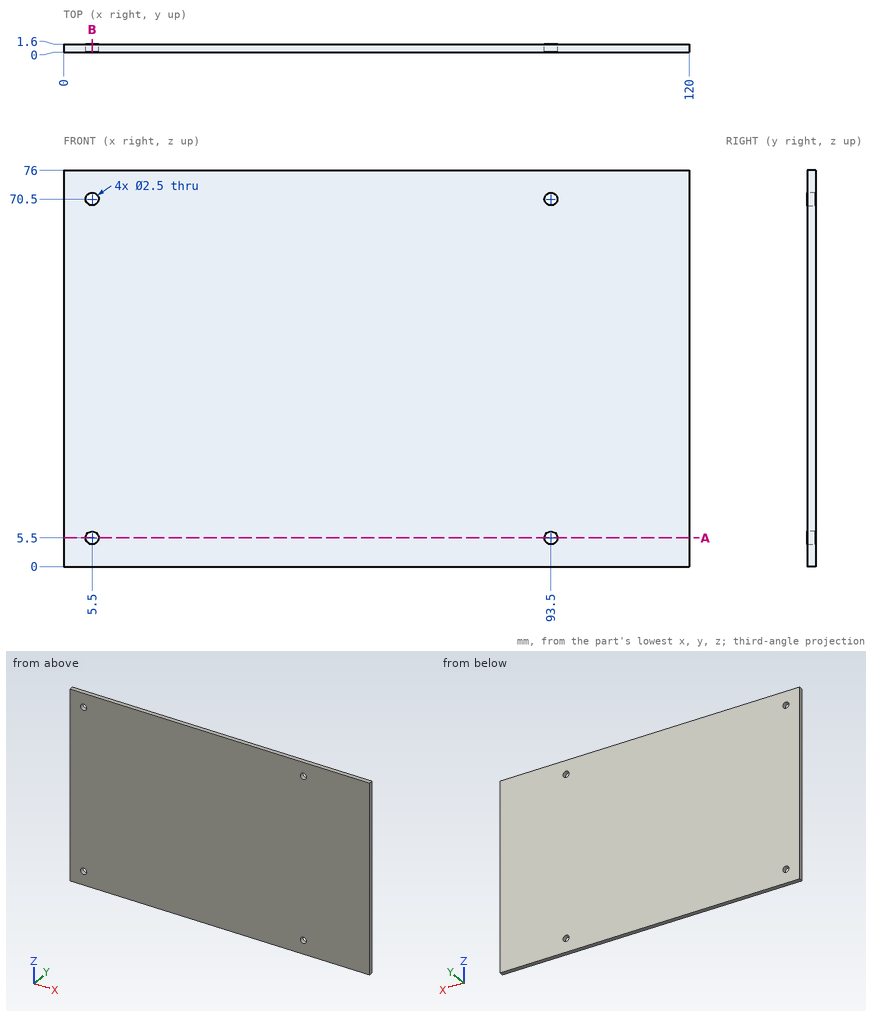
For this review, use the dimensioned drawing (mm, ordinates from the lowest corner) and the shaded views. Coordinates: 2 decimals unless noted, no trailing zeros. Loops run counter-clockwise (first coordinate to the right, second up) from the corner with the lowest first, then second, coordinate; pieces in that order, holes last. Notation, with made-up numbers: (89, 17) -> (111, 17) arc R23 cw to (111, 50) -> close; hole circle Ø9 at (20, -23.5). An arc over 180 degrees is marked (long way). Return JSON: item names as keys, results as strings. Group by question number.
(1) For pin 1 Ø1 at (x, z) = (14, 48.5) entering from -Y; pin 2 Ø2 at (x, z) = (5.5, 70.5) entering from -Y, all flat-tipped, find the tip position at first contact; note any pin that passes through.
(2) To check wall thickness, follow L1, parallel to X at y = 0.45, z = 70.5; L2, parallel to X at y = 0.75, z = 71.5. State the ranges of each line that lie inside material, in increasing order.
(3) Consider section B-B, the plane x = 5.5. Give the boundary of the cut face in (y, z).
(4) Consider section A-A, the plane z = 5.5. Give the boundary of the cut face in (x, y), plus the area to 3 significant figures.
Results below:
{
 "1": {"pin 1": "stops at y = 0", "pin 2": "passes through"},
 "2": {"L1": "x = 0 to 4.25, 6.75 to 92.25, 94.75 to 120", "L2": "x = 0 to 4.75, 6.25 to 92.75, 94.25 to 120"},
 "3": {"outline": "(0, 0) -> (1.6, 0) -> (1.6, 4.25) -> (0, 4.25) -> close; (0, 6.75) -> (1.6, 6.75) -> (1.6, 69.25) -> (0, 69.25) -> close; (0, 71.75) -> (1.6, 71.75) -> (1.6, 76) -> (0, 76) -> close"},
 "4": {"outline": "(0, 0) -> (4.25, 0) -> (4.25, 1.6) -> (0, 1.6) -> close; (6.75, 0) -> (92.25, 0) -> (92.25, 1.6) -> (6.75, 1.6) -> close; (94.75, 0) -> (120, 0) -> (120, 1.6) -> (94.75, 1.6) -> close", "area": "184 mm2"}
}
